For this review, use the dimensioned drawing (mm, ordinates from the lowest corner) and the shaded views. A direction names the side the tool comes from. Coordinates: 2 decimals unless noted, no trailing zeros. Write each loop counter-clockwise with the first axis right and the second up, starting at its lowest first coordinate (ties: lowest second). Pieces come first, ordered by that corner, then holes.
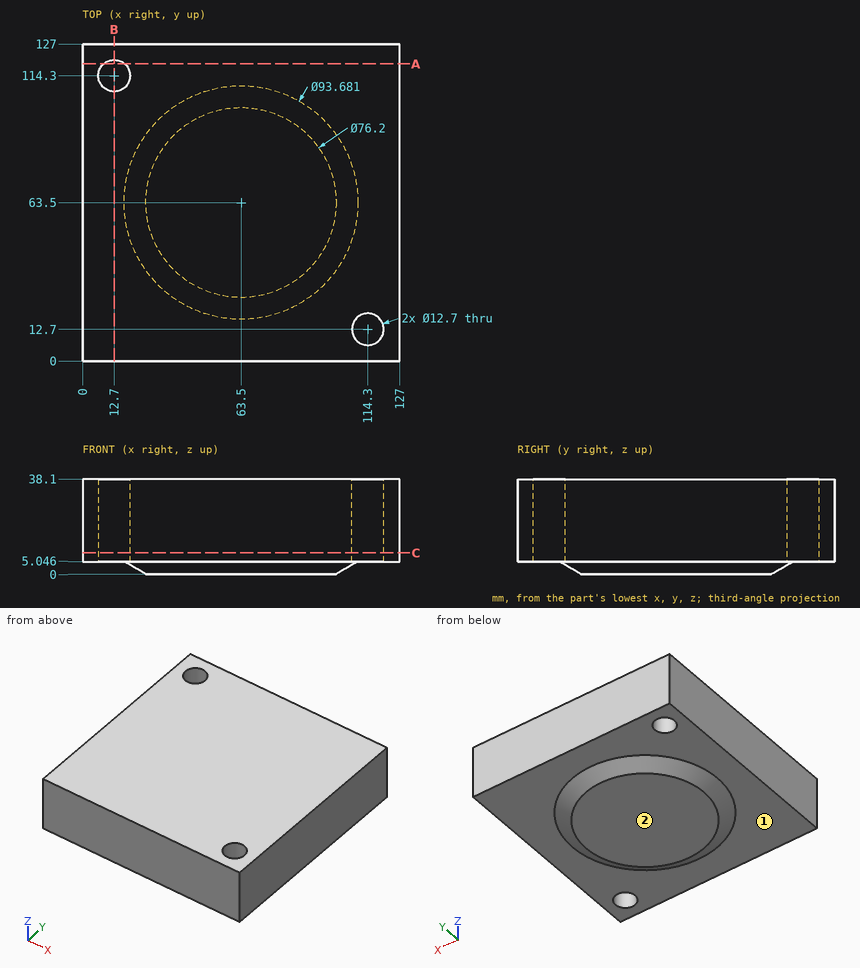
Item 1: To check wall thickness, follow line 1 along X through (y, z) = (114.3, 20); line 2 along Y through (x, z) = (12.7, 16). State the ranges of each line that lie inside material, in increasing order.
Solved:
line 1: x = 0 to 6.35, 19.05 to 127
line 2: y = 0 to 107.95, 120.65 to 127
Item 2: Take a section at A-A, the plane y = 119. Write out the cut boundary in (x, z), plus the area to 3 significant figures.
Solved:
outline: (0, 5.05) - (8.43, 5.05) - (8.43, 38.1) - (0, 38.1) - close; (16.97, 5.05) - (127, 5.05) - (127, 38.1) - (16.97, 38.1) - close
area: 3,920 mm2
Item 3: Machinability: for the marked faces 1 and 2, which of the approach directions +Z, -Z, +X, -X, +Y, -Y give a long, thin tool a straight path to every point of the face, cutting with its end or side? Answer none if there is none.
Solved:
face 1: -Z
face 2: -Z, +X, -X, +Y, -Y
Item 4: Take a section at C-C, the plane z = 8.5. Write out the cut boundary in (x, y), plus the area to 3 significant figures.
Solved:
outline: (0, 0) - (127, 0) - (127, 127) - (0, 127) - close; hole circle Ø12.7 at (12.7, 114.3); hole circle Ø12.7 at (114.3, 12.7)
area: 15,900 mm2
Item 5: For pin 1 (16.5 mm diameter, centred on x = 114.3, y = 12.7, fed in from -Z), flat-tipped, find the tip position at first contact; note if it passes through.
Solved:
pin 1: stops at z = 5.05
Item 6: Take a section at B-B, the plane x = 12.7. Write out the cut boundary in (y, z), plus the area to 3 significant figures.
Solved:
outline: (0, 5.05) - (107.95, 5.05) - (107.95, 38.1) - (0, 38.1) - close; (120.65, 5.05) - (127, 5.05) - (127, 38.1) - (120.65, 38.1) - close
area: 3,780 mm2
